```python
from build123d import *

# Parameters (mm, degrees)
F0_R     = 50.8
F0_R_2   = 1.5875
F1_DEPTH = 25.4
F2_DEPTH = 25.4
F3_R     = 5.08


with BuildPart() as f1:
    # F0 (on Top) → F1 (new body)
    with BuildSketch(Plane.XY):
        Circle(F0_R)
        Circle(F0_R_2, mode=Mode.SUBTRACT)
    extrude(amount=F1_DEPTH)

    # F0 (on Top) → F2 (join)
    with BuildSketch(Plane.XY):
        Circle(F0_R)
        Circle(F0_R_2, mode=Mode.SUBTRACT)
    extrude(amount=F2_DEPTH)

    # F3
    f3_edges = [f1.edges().sort_by_distance(p)[0] for p in [
        (-50.8, 0, 0),
        (50.8, 0, 12.7),
        (-50.8, 0, 25.4),
    ]]
    fillet(f3_edges, radius=F3_R)


solid = f1.part
```
CAD build for the part. Positions are in the model's coordinates, mm. Round coordinates to 2 decimals unless told otherwise and drop trailing zeros. Write each loop counter-clockwise with the first axis right and the second up, starting at its lowest first coordinate (ties: lowest second). Pieces come first, ordered by that corner, then holes. Notation, with made-up numbers: M 26,-9 L 53,-9 A19 cw 53,2 Z; hole C 52,21.25 d9. An arc over 180 degrees is marked long. One line per question, with ' | ' between items.
1. Pin check, flat tips, straight feed: pin 1 Ø4 at (x, z) = (-39, 5.5) entering from -Y; pin 2 Ø10 at (x, z) = (-39, 12) entering from -Y; pin 3 Ø5 at (x, y) = (19.5, -16) entering from -Z; pin 4 Ø5 at (x, z) = (-20.5, 10) entering from -Y. Stop position of each tip, or through.
Working result:
pin 1: y = -34.81 | pin 2: y = -37.74 | pin 3: z = 0 | pin 4: y = -47.5
2. Probe L1, parallel to Y at x = 0, z = 5.5; L2, parallel to X at y = 33.5, z = 15.5; L3, parallel to Y at x = 11, z = 2.5. List the from-to ranges inside material, lowest first. Write a range as from..to.
Working result:
L1: -50.8..-1.59, 1.59..50.8 | L2: -38.19..38.19 | L3: -48.87..48.87
3. Cut at C-C on z = 18.25. Write the cut outline in (x, y) (1 decimal).
Working result:
outline: C 0,0 d101.6; hole C 0,0 d3.2
4. Cut at D-D on z = 3. Write the cut outline in (x, y) (1 decimal), and give its area (3 significant figures).
Working result:
outline: C 0,0 d100.7; hole C 0,0 d3.2 | area: 7,960 mm2
5. Cut at A-A on x = 0. Write the cut outline in (y, z).
Working result:
outline: M -50.8,5.08 A5.08 ccw -45.72,0 L -1.59,0 L -1.59,25.4 L -45.72,25.4 A5.08 ccw -50.8,20.32 Z; M 1.59,0 L 45.72,0 A5.08 ccw 50.8,5.08 L 50.8,20.32 A5.08 ccw 45.72,25.4 L 1.59,25.4 Z
6. Mould opens along X. For faces 1 (the flat face through (-1, -10, 25.4)), 2 (the cylindrical face through (-11.012, -49.592, 12.593)), 3 (the cylindrical face through (-0.34, -1.55, 12.52)) say: pulls with the +X half, pulls with the -X half, needs draft (parallel to the pull), parting line crosses it, or undercut.
Working result:
face 1: needs draft | face 2: parting line crosses it | face 3: undercut
